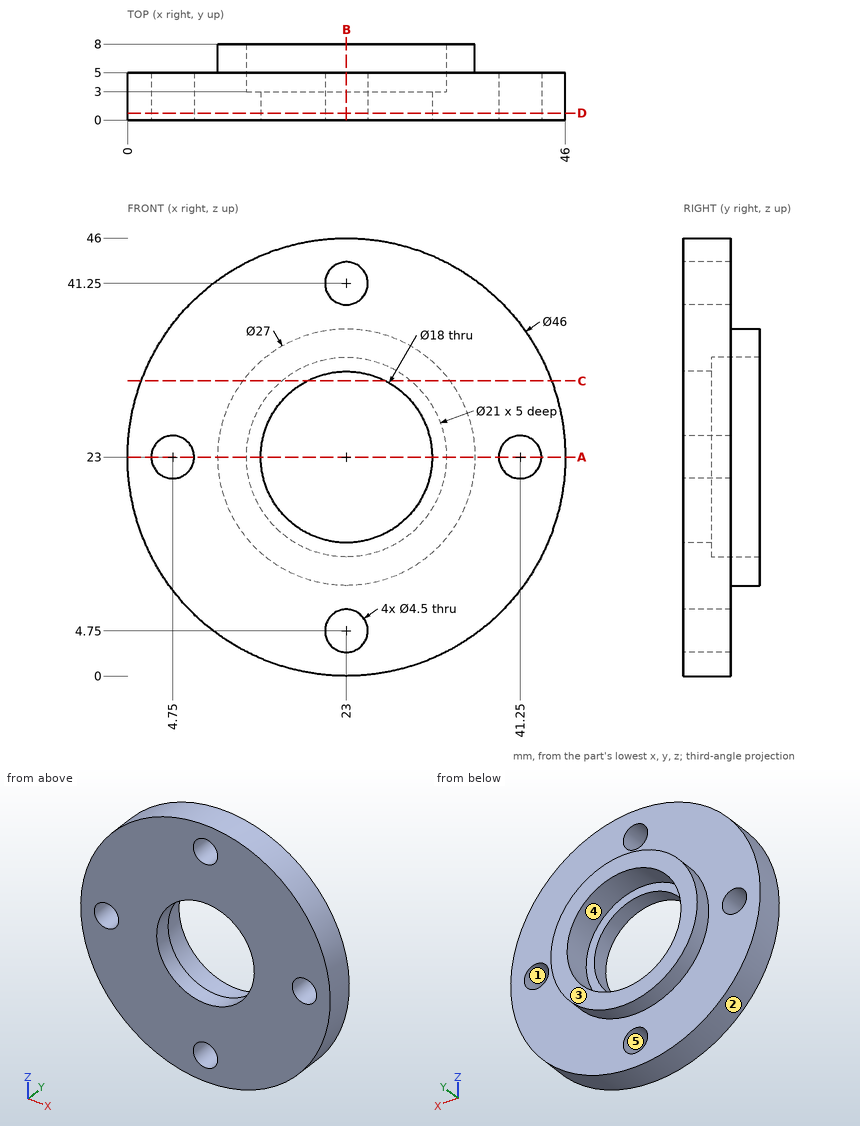
Job drawing, mm, ordinate dimensions from the low corner. One solid piece. A direction names the side the tool comes from. Round coordinates to 2 decimals unless told otherwise and drop trailing zeros. Write each loop counter-clockwise with the first axis right and the second up, starting at its lowest first coordinate (ties: lowest second). Pieces come first, ordered by that corner, then holes. Notation, with made-up numbers: M -0.75,62.5 L 7.25,62.5 A23 cw 7.25,84.5 Z; hole C 20.5,14.5 d2. An arc over 180 degrees is marked long. Return JSON: item names as keys, results as strings. Group by question number.
(1) Saw through at B-B on x = 23. Write the cut outline in (y, z), then the cut area to 3 significant figures.
(2) Pin check, flat tips, straight feed: pin 1 Ø19 at (x, z) = (23, 23) entering from +Y; pin 2 Ø7 at (x, z) = (4.75, 23) entering from +Y; pin 3 Ø3 at (y, z) = (4.5, 39) entering from +X. Stop position of each tip, or through.
(3) Saw through at A-A on z = 23. Write the cut outline in (x, y), then the cut area to 3 significant figures.
(4) Saw through at C-C on z = 31. Write the cut outline in (x, y), then the cut area to 3 significant figures.
(5) Which spindle directions (+Z, -Z, +X, -X, +Y, -Y) get a long thin tool onto all of the face, cutting with end or side? Do the marked faces 4 and 5. Say none if no direction does.
(6) Saw through at D-D on y = 0.75. Write the cut outline in (x, z), then the cut area to 3 significant figures.
(7) Two-plate mould, pull along X, no slides. Class the marked faces 1, 2 and 3: +X half, -X half, draft (parallel to the pull), parting line (faces both ways), or undercut.
(8) Drill centre lines: probe 1 along Y at (x, z) = (11, 42.5); probe 2 along X at (y, z) = (1, 26); probe 3 along X at (y, z) = (2.4, 41.25). Where is each one in solid material? Low to high.
Returned:
{
 "1": {"outline": "M 0,0 L 5,0 L 5,2.5 L 0,2.5 Z; M 0,7 L 5,7 L 5,9.5 L 8,9.5 L 8,12.5 L 3,12.5 L 3,14 L 0,14 Z; M 0,32 L 3,32 L 3,33.5 L 8,33.5 L 8,36.5 L 5,36.5 L 5,39 L 0,39 Z; M 0,43.5 L 5,43.5 L 5,46 L 0,46 Z", "area": "107 mm²"},
 "2": {"pin 1": "y = 3", "pin 2": "y = 5", "pin 3": "x = 40.85"},
 "3": {"outline": "M 0,0 L 2.5,0 L 2.5,5 L 0,5 Z; M 7,0 L 14,0 L 14,3 L 12.5,3 L 12.5,8 L 9.5,8 L 9.5,5 L 7,5 Z; M 32,0 L 39,0 L 39,5 L 36.5,5 L 36.5,8 L 33.5,8 L 33.5,3 L 32,3 Z; M 43.5,0 L 46,0 L 46,5 L 43.5,5 Z", "area": "107 mm²"},
 "4": {"outline": "M 1.44,0 L 18.88,0 L 18.88,3 L 16.2,3 L 16.2,8 L 12.13,8 L 12.13,5 L 1.44,5 Z; M 27.12,0 L 44.56,0 L 44.56,5 L 33.87,5 L 33.87,8 L 29.8,8 L 29.8,3 L 27.12,3 Z", "area": "188 mm²"},
 "5": {"face 4": "+Y", "face 5": "+Y, -Y"},
 "6": {"outline": "C 23,23 d46; hole C 4.75,23 d4.5; hole C 23,23 d18; hole C 23,4.75 d4.5; hole C 23,41.25 d4.5; hole C 41.25,23 d4.5", "area": "1,340 mm²"},
 "7": {"face 1": "undercut", "face 2": "parting line", "face 3": "draft"},
 "8": {"probe 1": "0 to 5", "probe 2": "0.2 to 14.51, 31.49 to 45.8", "probe 3": "9 to 20.75, 25.25 to 37"}
}
